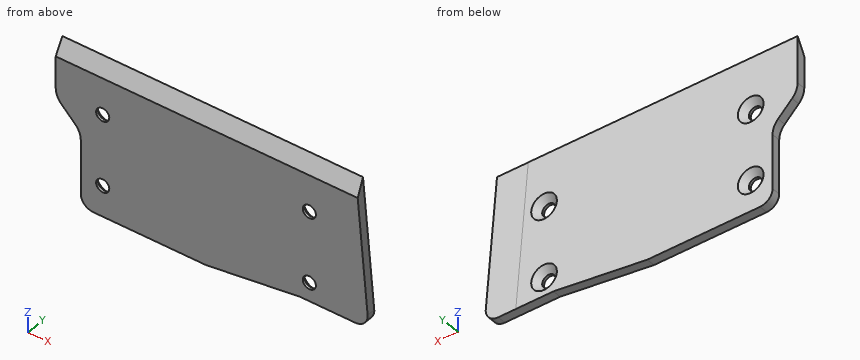
```python
from build123d import *

# Parameters (mm, degrees)
BOSS_EXTRUDE1_DEPTH = 2.8
CHAMFER1_SIZE       = 3
CHAMFER1_SIZE_2     = 5.196152423
SKETCH2_R           = 2.1
CUT_EXTRUDE1_DEPTH  = 103.74283559
CHAMFER2_SIZE       = 2
FILLET1_R           = 6
FILLET2_R           = 4
CUT_EXTRUDE2_DEPTH  = 0.01


with BuildPart() as part:
    # Sketch1 → Boss-Extrude1 (new body)
    with BuildSketch(Plane(origin=(0, 0, 0), x_dir=(1, 0, 0), z_dir=(0, 1, 0))):
        Polygon((0, 4), (40, 4), (70, 0), (92, 0), (88, -46), (0, -46), (-8, -46), (-8, -28), (0, -20), align=None)
    extrude(amount=BOSS_EXTRUDE1_DEPTH)

    # Chamfer1
    # the kernel refuses this chamfer: 5.196152423, 3 mm, written as the material it takes off along each edge
    with BuildSketch(Plane(origin=(-21.442891912, 0, 46), x_dir=(0, 0.9983227437537926, 0.05789386240267091), z_dir=(1, 0, 0))) as chamfer1_piece_1:
        Polygon((CHAMFER1_SIZE * 0.998322743754, -CHAMFER1_SIZE * 0.0578938624027), (-CHAMFER1_SIZE_2 * 0.0578938623994, -CHAMFER1_SIZE_2 * 0.998322743697), (0, 0), align=None)
    extrude(amount=122.885783824, mode=Mode.SUBTRACT)

    # Sketch2 → Cut-Extrude1 (cut, through all)
    with BuildSketch(Plane(origin=(0, 2.8, 0), x_dir=(1, 0, 0), z_dir=(0, 1, 0))):
        with Locations(Location((7, -6, 0), (0, 0, 270))):
            Circle(SKETCH2_R)
        with Locations(Location((7, -29, 0), (0, 0, 270))):
            Circle(SKETCH2_R)
        with Locations(Location((73, -6, 0), (0, 0, 270))):
            Circle(SKETCH2_R)
        with Locations(Location((73, -29, 0), (0, 0, 270))):
            Circle(SKETCH2_R)
    extrude(amount=-CUT_EXTRUDE1_DEPTH, mode=Mode.SUBTRACT)

    # Chamfer2
    chamfer2_edges = [part.edges().sort_by_distance(p)[0] for p in [
        (7, 2.8, 26.9),
        (73, 2.8, 3.9),
        (73, 2.8, 26.9),
        (7, 2.8, 3.9),
    ]]
    chamfer(chamfer2_edges, length=CHAMFER2_SIZE)

    # Fillet1
    fillet1_edges = [part.edges().sort_by_distance(p)[0] for p in [
        (-8, 1.4, 28),
        (0, 1.4, 20),
    ]]
    fillet(fillet1_edges, radius=FILLET1_R)

    # Fillet2
    fillet2_edges = [part.edges().sort_by_distance(p)[0] for p in [
        (0, 1.4, -4),
        (92, 1.4, 0),
    ]]
    fillet(fillet2_edges, radius=FILLET2_R)

    # Sketch3 → Cut-Extrude2 (cut)
    with BuildSketch(Plane(origin=(0, 2.8, 0), x_dir=(1, 0, 0), z_dir=(0, 1, 0))):
        Polygon((78.041306422, -45.653589838), (82.011183799, 0), (92.341682138, 0.80141962), (88.030122623, -45.653589838), align=None)
    extrude(amount=-CUT_EXTRUDE2_DEPTH, mode=Mode.SUBTRACT)


solid = part.part
```
Read the model definition and answer for the solid it produces. Units are mm, in the model's axes. Coordinates: 2 decimals unless noted, no trailing zeros. Loops run counter-clockwise (first coordinate to the right, second up) from the corner with the lowest first, then second, coordinate; pieces in that order, holes last. Notation, with made-up numbers: (52, 83.5) - (80, 83.5) arc R25 cw to (80, 104.5) - close; hole circle Ø8 at (52, 25). An arc over 180 degrees is marked (long way). Answer in a Markdown table with one row per item.
1. Find section B-B, the plane y = 1.3. Write down the section's boundary in (x, z).
Conclusion:
| item | result |
|---|---|
| outline | (-8, 30.49) arc R6 ccw to (-6.24, 26.24) - (-1.76, 21.76) arc R6 cw to (0, 17.51) - (0, 0) arc R4 ccw to (4, -4) - (40, -4) - (70, 0) - (87.64, 0) arc R4 ccw to (91.62, 4.35) - (88.26, 43.06) - (-8, 43.06) - close; hole circle Ø5.2 at (7, 6); hole circle Ø5.2 at (7, 29); hole circle Ø5.2 at (73, 6); hole circle Ø5.2 at (73, 29) |
2. Given pin 1 (3.5 mm diameter, centred on x = 7, z = 6, fed in from +Y); pin 2 (5 mm diameter, centred on x = 73, z = 6, fed in from -Y), each flat-ended and moving along its own axis, determine where each tip first touches the part or whether it passes through.
Conclusion:
| item | result |
|---|---|
| pin 1 | passes through |
| pin 2 | stops at y = 0 |
3. Straight lines are drawn through the part: line 1 (X direction, y = 0.2, z = 6); line 2 (Z direction, x = 75, y = 2.7); line 3 (X direction, y = 1.55, z = 4). For each, find the intervals that lie inside material, in ascending order.
Conclusion:
| item | result |
|---|---|
| line 1 | x = 0 to 4.9, 9.1 to 70.9, 75.1 to 91.48 |
| line 2 | z = 0 to 2.54, 9.46 to 25.54, 32.46 to 45.48 |
| line 3 | x = 0 to 4.97, 9.03 to 70.97, 75.03 to 91.64 |
4. Find section A-A, the plane x = 73. Write down the section's boundary in (y, z).
Conclusion:
| item | result |
|---|---|
| outline | (0, 0) - (2.8, 0) - (2.8, 1.9) - (0.8, 3.9) - (0, 3.9) - close; (0, 8.1) - (0.8, 8.1) - (2.8, 10.1) - (2.8, 24.9) - (0.8, 26.9) - (0, 26.9) - close; (0, 31.1) - (0.8, 31.1) - (2.8, 33.1) - (2.8, 45.65) - (0, 40.8) - close |
5. Find section C-C, the plane z = 29. Count the separate pieces of the cut face and the enclosed holes in it, then the cut area to 3 significant figures.
Conclusion:
| item | result |
|---|---|
| separate pieces | 3 |
| enclosed holes | 0 |
| area | 241 mm² |
6. Find section D-D, the plane x = 26. Write down the section's boundary in (y, z).
Conclusion:
| item | result |
|---|---|
| outline | (0, -4) - (2.8, -4) - (2.8, 45.65) - (0, 40.8) - close |
